from build123d import *

# Parameters (mm, degrees)
F0_W     = 0.1549944282
F0_H     = 44.9563041329
F0_W_2   = 3.2087042928
F0_W_3   = 145.5950886011
F0_H_2   = 107.2087809443
F0_W_4   = 3.4092515707
F0_W_5   = 0.1821219921
F0_H_3   = 107.1085110307
F1_DEPTH = 25.4
F3_DEPTH = 2.54


with BuildPart() as f1:
    # F0 (on Front) → F1 (new body)
    with BuildSketch(Plane.XZ):
        with Locations((-76.1510320008, 53.7468977273)):
            Rectangle(F0_W, F0_H)
        with Locations((-74.4691826403, 53.7468977273)):
            Rectangle(F0_W_2, F0_H)
        with Locations((-0.0672861934, 53.7468977273)):
            Rectangle(F0_W_3, F0_H)
        with Locations((-74.4691826403, -22.3356448114)):
            Rectangle(F0_W_2, F0_H_2)
        with Locations((74.4348838925, 53.7468977273)):
            Rectangle(F0_W_4, F0_H)
        with Locations((76.2305706739, 53.7468977273)):
            Rectangle(F0_W_5, F0_H)
        with Locations((74.4348838925, -22.2855098546)):
            Rectangle(F0_W_4, F0_H_3)
    extrude(amount=F1_DEPTH)

    # F2 (on face) → F3 (join)
    with BuildSketch(Plane.XZ.offset(25.4)):
        Polygon((-36.8280895054, 59.82850492), (-36.8280895054, 44.7937846184), (-24.8050373048, 44.6476303041), (-24.8050373048, 59.82850492), align=None)
        Polygon((-47.2566857934, 59.0478740633), (-62.004558742, 58.6273260415), (-62.004558742, 43.9759418368), (-47.2566857934, 43.9759418368), align=None)
    extrude(amount=F3_DEPTH)


solid = f1.part
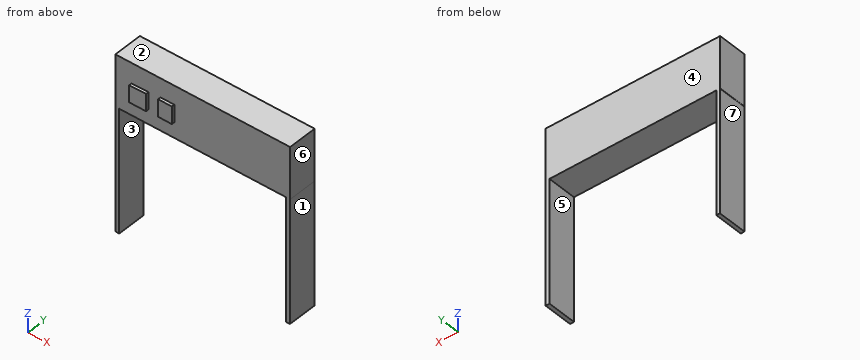
Geometry: final body of the model. Coordinates: model frame, mm. Face numbers are marked on the shaded views. A direction names the side the tool comes from. Round coordinates to 2 decimals unless told otherwise and drop trailing zeros. Loops run counter-clockwise (first coordinate to the right, second up) from the corner with the lowest first, then second, coordinate; pieces in that order, holes last.
Q1. Section C-C on z = 55. Return loops of the section in (x, y).
Q2. Pin query (flat end, axial travel): P1, Ø2, axis at y = -27, z = 51, coming from the +X side; P2, Ø1.5, axis at x = 54, y = -17.5, coming from the -Z side; P3, Ø12, axis at y = -14.5, z = -6, coming from the +X side. Return the tip coordinate at first contact, or that it passes through.
Q3. Material intervals for L1, parallel to X at y = -8.5, z = 20; L2, parallel to Y at x = 12, z = 31.5; L3, parallel to Z at x = -7.5, y = -21, sorted ascending.
Q4. Section D-D on x = 32. Return loops of the section in (y, z).
Q5. Pull-direction query (X, two-part tool) for the marked faces 4, 5, 6 and 7; classes: released by +X, released by -X, zero draft, split by the parting line, or undercut.
Q6. Access query for the marked faces 1, 2 and 3. Directions: +Z, -Z, +X, -X, +Y, -Y. A direction counts if a zero-diameter tool reaches every point of the face in a straight line with its end or side. Return the directions, or none.
Q7. Section B-B on y = -10. Return loops of the section in (x, z), plus the area to 3 significant figures.
Q8. Section A-A on z = -3.5. Return loops of the section in (x, y), plus the area to 3 significant figures.
Evaluation:
1. outline: (-76.23, -25.4) - (-62, -25.4) - (-62, -27.94) - (-47.26, -27.94) - (-47.26, -25.4) - (-36.83, -25.4) - (-36.83, -27.94) - (-24.81, -27.94) - (-24.81, -25.4) - (76.32, -25.4) - (76.32, 0) - (-76.23, 0) - close
2. P1: stops at x = -24.81
2. P2: stops at z = 31.27
2. P3: stops at x = 76.14
3. L1: x = -76.07 to -72.86, 72.73 to 76.14
3. L2: y = -25.4 to 0
3. L3: z = 31.27 to 76.23
4. outline: (-25.4, 31.27) - (0, 31.27) - (0, 76.23) - (-25.4, 76.23) - close
5. face 4: zero draft
5. face 5: undercut
5. face 6: released by +X
5. face 7: released by -X
6. face 1: -Z, +X, +Y, -Y
6. face 2: +Z, +X, -X, +Y, -Y
6. face 3: -Z, +Y, -Y
7. outline: (-76.23, 31.27) - (-76.07, 31.27) - (-76.07, -75.94) - (-72.86, -75.94) - (-72.86, 31.27) - (72.73, 31.27) - (72.73, -75.84) - (76.14, -75.84) - (76.14, 31.27) - (76.32, 31.27) - (76.32, 76.23) - (-76.23, 76.23) - close
7. area: 7,570 mm2
8. outline: (-76.07, -25.4) - (-72.86, -25.4) - (-72.86, 0) - (-76.07, 0) - close; (72.73, -25.4) - (76.14, -25.4) - (76.14, 0) - (72.73, 0) - close
8. area: 168 mm2
